```python
from build123d import *

# Parameters (mm, degrees)
F0_W     = 206.1464
F0_H     = 89.435898
F1_DEPTH = 10.16
F2_T     = -6.35
F3_W     = 88.9
F3_H     = 66.04
F4_DEPTH = 3.81


with BuildPart() as f1:
    # F0 (on Front) → F1 (new body)
    with BuildSketch(Plane.XZ):
        Rectangle(F0_W, F0_H)
    extrude(amount=F1_DEPTH)

    # F2
    f2_openings = [f1.faces().sort_by_distance(p)[0] for p in [
        (0, -10.16, 0),
    ]]
    offset(amount=F2_T, openings=f2_openings)

    # F3 (on face) → F4 (join, through all)
    with BuildSketch(Plane.XZ.offset(6.35)):
        with Locations((0, 5.347949)):
            Rectangle(F3_W, F3_H)
    extrude(amount=F4_DEPTH)


solid = f1.part
```
Geometry check sheet. Reference: the model listing, model coordinates, mm. A direction names the side the tool comes from. Round coordinates to 2 decimals unless told otherwise and drop trailing zeros. Loops run counter-clockwise (first coordinate to the right, second up) from the corner with the lowest first, then second, coordinate; pieces in that order, holes last. Notation, with made-up numbers: (-28.75, 27.25) -> (25.25, 27.25) arc R18 cw to (25.25, 41.25) -> close; hole circle Ø10 at (2, 33). An arc over 180 degrees is marked (long way). Use a Markdown table: item, result.
(1) Scan lines: probe 1 along X at (y, z) = (-6.5, 12.5); probe 2 along Z at (x, y) = (-66, -7); probe 3 along Z at (x, y) = (-40, -8.25). Record each from-to range of solid material in increasing order.
Calculated:
| item | result |
|---|---|
| probe 1 | -103.07 to -96.72, -44.45 to 44.45, 96.72 to 103.07 |
| probe 2 | -44.72 to -38.37, 38.37 to 44.72 |
| probe 3 | -44.72 to -38.37, -27.67 to 44.72 |
(2) Sectioned sample at D-D (x = -20). Enter the section's corners in (y, z), then the cut area to 3 significant figures.
Calculated:
| item | result |
|---|---|
| outline | (-10.16, -44.72) -> (0, -44.72) -> (0, 44.72) -> (-10.16, 44.72) -> (-10.16, -27.67) -> (-6.35, -27.67) -> (-6.35, -38.37) -> (-10.16, -38.37) -> close |
| area | 868 mm² |
(3) Sectioned sample at B-B (x = -54.5). Enter the section's corners in (y, z), then the cut area to 3 significant figures.
Calculated:
| item | result |
|---|---|
| outline | (-10.16, -44.72) -> (0, -44.72) -> (0, 44.72) -> (-10.16, 44.72) -> (-10.16, 38.37) -> (-6.35, 38.37) -> (-6.35, -38.37) -> (-10.16, -38.37) -> close |
| area | 616 mm² |
(4) Sectioned sample at A-A (y = -8.5). Enter the section's corners in (x, z).
Calculated:
| item | result |
|---|---|
| outline | (-103.07, -44.72) -> (103.07, -44.72) -> (103.07, 44.72) -> (-103.07, 44.72) -> close; hole (-96.72, -38.37) -> (96.72, -38.37) -> (96.72, 38.37) -> (44.45, 38.37) -> (44.45, -27.67) -> (-44.45, -27.67) -> (-44.45, 38.37) -> (-96.72, 38.37) -> close |
(5) Mould release check, pull along X, two halves, no side actions. Record for faces 1 (the flat face through (-1, 0, 1)), 2 (the flat face through (103.073, -5, -1)), 3 (the flat face through (-1, -6.35, -34)): released by +X, released by -X, zero draft, split by the parting line, or undercut.
Calculated:
| item | result |
|---|---|
| face 1 | zero draft |
| face 2 | released by +X |
| face 3 | undercut |
(6) Sectioned sample at C-C (z = 4.5). Enter the section's corners in (x, y), then the cut area to 3 significant figures.
Calculated:
| item | result |
|---|---|
| outline | (-103.07, -10.16) -> (-96.72, -10.16) -> (-96.72, -6.35) -> (-44.45, -6.35) -> (-44.45, -10.16) -> (44.45, -10.16) -> (44.45, -6.35) -> (96.72, -6.35) -> (96.72, -10.16) -> (103.07, -10.16) -> (103.07, 0) -> (-103.07, 0) -> close |
| area | 1,700 mm² |
(7) Go/stop test with a flat-tipped pin: P1, Ø6, axis at x = 52, z = 24.5, coming from the -Y side. Record where the tip stops, or that it passes through.
Calculated:
| item | result |
|---|---|
| P1 | y = -6.35 |
(8) Set-up check for faces 4 (the flat face through (-71, -8, 38.368)), 5 (the flat face through (-1, -5, -44.718)): record each of +Z, -Z, +X, -X, +Y, -Y from which the full face is reachable in a straight line by a thin tool's end or side.
Calculated:
| item | result |
|---|---|
| face 4 | -Y |
| face 5 | -Z, +X, -X, +Y, -Y |
